Source: CAD feature listing. Evaluate the final solid. Frame: model axes, mm. Face numbers are marked on the shaded views. Give positions to 0.01 mm unless a question says otherwise; leave off trailing zeros. Loops run counter-clockwise (first coordinate to the right, second up) from the corner with the lowest first, then second, coordinate; pieces in that order, holes last. Notation, with made-up numbers: M 71.5,18 L 107.5,18 A11 cw 107.5,34 Z; hole C -27.75,-17 d10. An arc over 180 degrees is marked long. Answer in a Markdown table with one row per item.
```python
from build123d import *

# Parameters (mm, degrees)
BOSS_EXTRUDE1_DEPTH = 1800
BOSS_EXTRUDE2_DEPTH = 1800
SHELL1_T            = -10
FILLET1_R           = 10
SKETCH3_R           = 10
CUT_EXTRUDE1_DEPTH  = 2134.346626248


with BuildPart() as part:
    # Sketch1 → Boss-Extrude1 (new body)
    with BuildSketch(Plane.XY):
        with BuildLine():
            Line((0, 0), (384.757529665, 0))
            ThreePointArc((384.757529665, 0), (502.844648307, 98.659137532), (620.931766949, 0))
            Line((620.931766949, 0), (1000, 0))
            ThreePointArc((1000, 0), (500, 500), (0, 0))
        make_face()
    extrude(amount=BOSS_EXTRUDE1_DEPTH)

    # Sketch2 → Boss-Extrude2 (add)
    with BuildSketch(Plane.XY):
        Polygon((1000, 0), (1039.599839872, 0), (1039.599839872, 20), (999.599839872, 20), align=None)
        Polygon((0, 0), (-39.599839872, 0), (-39.599839872, 20), (0.400160128, 20), align=None)
    extrude(amount=BOSS_EXTRUDE2_DEPTH)

    # Shell1
    shell1_openings = [part.faces().sort_by_distance(p)[0] for p in [
        (830.265803411, 0, 900),
        (502.844648307, 98.659137532, 900),
        (172.578844897, 0, 900),
    ]]
    offset(amount=SHELL1_T, openings=shell1_openings, kind=Kind.INTERSECTION)

    # Fillet1
    fillet1_edges = [part.edges().sort_by_distance(p)[0] for p in [
        (500, 500, 0),
        (500, 500, 1800),
    ]]
    fillet(fillet1_edges, radius=FILLET1_R)

    # Sketch3 → Cut-Extrude1 (cut, through all)
    with BuildSketch(Plane(origin=(0, 20, 0), x_dir=(1, 0, 0), z_dir=(0, 1, 0))):
        with Locations(Location((-18.235719302, -19.68953089, 0), (0, 0, 180))):
            Circle(SKETCH3_R)
        with Locations(Location((1021.817467904, -29.68953089, 0), (0, 0, 180))):
            Circle(SKETCH3_R)
        with Locations(Location((1021.817467904, -1751.208740349, 0), (0, 0, 180))):
            Circle(SKETCH3_R)
        with Locations(Location((-18.235719302, -1741.208740349, 0), (0, 0, 180))):
            Circle(SKETCH3_R)
    extrude(amount=-CUT_EXTRUDE1_DEPTH, mode=Mode.SUBTRACT)


solid = part.part
```
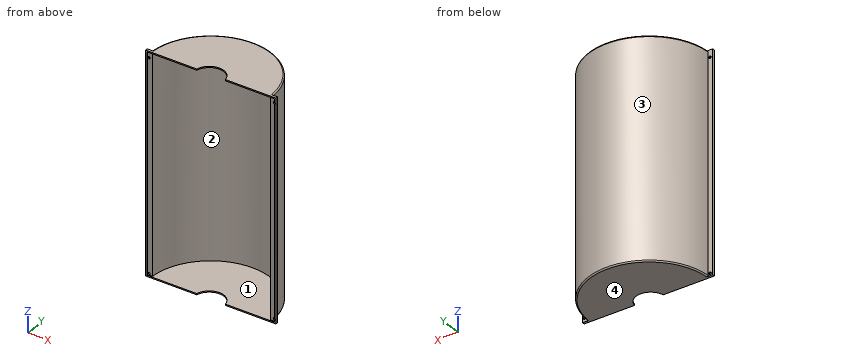
Q1. Ray query, probe 1 along Z at (x, y) = (658, 225.5); probe 2 along X at (y, z) = (153, 1060); probe 3 along X at (y, z) = (317, 273.5). Return the intervals inside material, ascending. Write a range as from..to.
Values follow:
| item | result |
|---|---|
| probe 1 | 0..10, 1790..1800 |
| probe 2 | 23.98..34.5, 965.5..976.02 |
| probe 3 | 113.33..126.35, 873.65..886.67 |
Q2. Mould query, pull axis X, two halves, no side actions, for the marked faces 1, 2, 3 and 4. Classes: +X half, -X half, draft (parallel to the pull), parting line (faces both ways), or undercut.
Values follow:
| item | result |
|---|---|
| face 1 | undercut |
| face 2 | undercut |
| face 3 | parting line |
| face 4 | draft |
Q3. Section query B-B (x = 500). Output: boundary loops of the cut face in (y, z).
Values follow:
| item | result |
|---|---|
| outline | M 98.63,0 L 490,0 A10 ccw 500,10 L 500,1790 A10 ccw 490,1800 L 98.63,1800 L 98.63,1790 L 490,1790 L 490,10 L 98.63,10 Z |
Q4. Contact query for flat-ended pins moving along their axis: pin 1 Ø12 at (x, z) = (1021.82, 1751.21) entering from +Y; pin 2 Ø20 at (x, z) = (-9, 1183) entering from -Y; pin 3 Ø10 at (x, z) = (443, 1519.5) entering from -Y; pin 4 Ø15 at (x, z) = (1025.5, 1017) entering from +Y. Output: stop coordinate, or through.
Values follow:
| item | result |
|---|---|
| pin 1 | through |
| pin 2 | y = 10 |
| pin 3 | y = 486.06 |
| pin 4 | y = 20 |
